Geometry check sheet. Reference: the model listing, model coordinates, mm. A direction names the side the tool comes from. Coordinates: 2 decimals unless noted, no trailing zeros. Loops run counter-clockwise (first coordinate to the right, second up) from the corner with the lowest first, then second, coordinate; pieces in that order, holes last. Notation, with made-up numbers: (41.25, 21) - (85.25, 21) arc R6 ccw to (85.25, 25) - close; hole circle Ø8 at (5, -17). An arc over 180 degrees is marked (long way). Write item = value, one per line. Start each with the question number.
from build123d import *

# Parameters (mm, degrees)
SKETCH1_W           = 120
SKETCH1_H           = 60
BOSS_EXTRUDE2_DEPTH = 80
SKETCH2_W           = 80
SKETCH2_H           = 10
CUT_EXTRUDE1_DEPTH  = 80
BOSS_EXTRUDE3_DEPTH = 80
SKETCH4_R           = 10
CUT_EXTRUDE2_DEPTH  = 80
CUT_EXTRUDE3_DEPTH  = 15
CUT_EXTRUDE4_DEPTH  = 45
CUT_EXTRUDE5_DEPTH  = 30
SKETCH13_W          = 80
SKETCH13_H          = 30
CUT_EXTRUDE12_DEPTH = 950
SKETCH14_W          = 10
SKETCH14_H          = 25
BOSS_EXTRUDE4_DEPTH = 30


with BuildPart() as part:
    # Sketch1 → Boss-Extrude2 (new body)
    with BuildSketch(Plane.XY):
        with Locations((60, 30)):
            Rectangle(SKETCH1_W, SKETCH1_H)
    extrude(amount=BOSS_EXTRUDE2_DEPTH)

    # Sketch2 → Cut-Extrude1 (cut)
    with BuildSketch(Plane.XY.offset(80)):
        with Locations((60, 5)):
            Rectangle(SKETCH2_W, SKETCH2_H)
    extrude(amount=-CUT_EXTRUDE1_DEPTH, mode=Mode.SUBTRACT)

    # Sketch3 → Boss-Extrude3 (add)
    with BuildSketch(Plane.XY.offset(80)):
        with BuildLine():
            Line((0, 60), (120, 60))
            ThreePointArc((120, 60), (60, 120), (0, 60))
        make_face()
    extrude(amount=-BOSS_EXTRUDE3_DEPTH)

    # Sketch4 → Cut-Extrude2 (cut)
    with BuildSketch(Plane.XY.offset(80)):
        with Locations((60, 60)):
            Circle(SKETCH4_R)
    extrude(amount=-CUT_EXTRUDE2_DEPTH, mode=Mode.SUBTRACT)

    # Sketch5 → Cut-Extrude3 (cut)
    with BuildSketch(Plane.XY.offset(80)):
        with BuildLine():
            Line((45, 80), (45, 118.094750193))
            ThreePointArc((45, 118.094750193), (60, 120.1113283), (75, 118.094750193))
            Line((75, 118.094750193), (75, 80))
            ThreePointArc((75, 80), (60, 35), (45, 80))
        make_face()
    extrude(amount=-CUT_EXTRUDE3_DEPTH, mode=Mode.SUBTRACT)

    # Sketch6 → Cut-Extrude4 (cut)
    with BuildSketch(Plane.XY.offset(80)):
        with BuildLine():
            Line((10, 30), (10, 60))
            ThreePointArc((10, 60), (12.565835097, 75.811388301), (20, 90))
            Line((20, 90), (20, 104.72135955))
            ThreePointArc((20, 104.72135955), (5.227744249, 84.494897428), (0, 60))
            Line((0, 60), (0, 30))
            Line((0, 30), (10, 30))
        make_face()
        with BuildLine():
            Line((100, 104.72135955), (100, 90))
            ThreePointArc((100, 90), (107.434164903, 75.811388301), (110, 60))
            Line((110, 60), (110, 30))
            Line((110, 30), (120, 30))
            Line((120, 30), (120, 60))
            ThreePointArc((120, 60), (114.772255751, 84.494897428), (100, 104.72135955))
        make_face()
    extrude(amount=-CUT_EXTRUDE4_DEPTH, mode=Mode.SUBTRACT)

    # Sketch7 → Cut-Extrude5 (cut)
    with BuildSketch(Plane.XY.offset(80)):
        with BuildLine():
            Line((0, 60), (10, 60))
            ThreePointArc((10, 60), (60, 110), (110, 60))
            Line((110, 60), (120, 60))
            ThreePointArc((120, 60), (60, 120), (0, 60))
        make_face()
    extrude(amount=-CUT_EXTRUDE5_DEPTH, mode=Mode.SUBTRACT)

    # Sketch13 → Cut-Extrude12 (cut)
    with BuildSketch(Plane(origin=(0, 10, 0), x_dir=(-1, 0, 0), z_dir=(0, -1, 0))):
        with Locations((-60, -35)):
            Rectangle(SKETCH13_W, SKETCH13_H)
    extrude(amount=-CUT_EXTRUDE12_DEPTH, mode=Mode.SUBTRACT)

    # Sketch14 → Boss-Extrude4 (add)
    with BuildSketch(Plane.XY.offset(20)):
        with Locations((60, 22.5)):
            Rectangle(SKETCH14_W, SKETCH14_H)
    extrude(amount=BOSS_EXTRUDE4_DEPTH)


solid = part.part
(1) Sectioned sample at D-D on z = 56.5. Enter the section's corners in (x, y).
(2) Tool access check on faces 1 (the face through (5, 30, 58)), 2 (the face through (65, 22, 35)), 3 (the face through (60, 35, 35)), 4 (the face through (60.874, 35.015, 72.605)). Record the directions out of +Z, -Z, +X, -X, +Y, -Y that give a thin tool (end or side, any length) a straight path to the whole face; none if there is none.
(3) Sectioned sample at A-A on z = 27.5. Enter the section's corners in (x, y), plus the area to 3 significant figures.
(4) Sectioned sample at B-B on y = 45. Enter the section's corners in (x, z), plus the area to 3 significant figures.
(5) Scan lines: line 1 (Z direction, x = 67, y = 44.5); line 2 (Y direction, x = 60, z = 55); line 3 (Z direction, x = 91.5, y = 14.5). Record each from-to range of solid material in increasing order.
(6) Draft check along X on faces 5 (the face through (100, 40, 41)), 6 (the face through (60, 73, 65)), 7 (the face through (10, 45, 58)), 8 (the face through (59, 48, 0)). Enter one of: pulls with the +X half, pulls with the -X half, needs draft (parallel to the pull), parting line crosses it, or undercut.
(7) Depth check by flat-ended pin: pin 1 (24 mm diameter, centred on y = 51.5, z = 61.5, fed in from +X); pin 2 (16.5 mm diameter, centred on y = 97.5, z = 69, fed in from -X); pin 3 (15 mm diameter, centred on y = 43, z = 48, fed in from -X). Enter the tip coordinate at first touch or a pass-through.
(8) Sectioned sample at C-C on x = 60. Enter the section's corners in (y, z), plus the area to 4 significant figures.
Working result:
q1.outline = (0, 0) - (20, 0) - (20, 10) - (100, 10) - (100, 0) - (120, 0) - (120, 30) - (110, 30) - (110, 60) arc R50 ccw to (10, 60) - (10, 30) - (0, 30) - close; hole circle Ø20 at (60, 60)
q2.face_1 = +Z, -X, +Y
q2.face_2 = +Y, -Y
q2.face_3 = +Y
q2.face_4 = +Z
q3.outline = (0, 0) - (20, 0) - (20, 104.72) arc R60 ccw to (0, 60) - close; (55, 10) - (65, 10) - (65, 35) - (55, 35) - close; (100, 0) - (120, 0) - (120, 60) arc R60 ccw to (100, 104.72) - close
q3.area = 3,890 mm2
q4.outline = (0, 0) - (120, 0) - (120, 35) - (110, 35) - (110, 80) - (80, 80) - (80, 65) - (40, 65) - (40, 80) - (10, 80) - (10, 35) - (0, 35) - close; hole (20, 20) - (100, 20) - (100, 50) - (20, 50) - close
q4.area = 5,700 mm2
q5.line_1 = 0 to 20, 50 to 65
q5.line_2 = 10 to 50, 70 to 110
q5.line_3 = 0 to 20, 50 to 80
q6.face_5 = undercut
q6.face_6 = undercut
q6.face_7 = pulls with the -X half
q6.face_8 = needs draft
q7.pin_1 = 110
q7.pin_2 = 19.45
q7.pin_3 = 10
q8.outline = (10, 0) - (50, 0) - (50, 20) - (35, 20) - (35, 50) - (50, 50) - (50, 65) - (35, 65) - (35, 80) - (10, 80) - close; (70, 0) - (120, 0) - (120, 20) - (70, 20) - close; (70, 50) - (110, 50) - (110, 65) - (70, 65) - close
q8.area = 4,125 mm2
